Model file for the job. Use its own axes, mm. A direction names the side the tool comes from. Round coordinates to 2 decimals unless told otherwise and drop trailing zeros. Loops run counter-clockwise (first coordinate to the right, second up) from the corner with the lowest first, then second, coordinate; pieces in that order, holes last. Notation, with made-up numbers: M 42,80 L 50,80 A31 cw 50,113 Z; hole C -7.5,65.5 d10. An arc over 180 degrees is marked long. Answer in a Markdown table with one row per item.
from build123d import *

# Parameters (mm, degrees)
SKETCH1_W               = 55
SKETCH1_H               = 80
BOSS_EXTRUDE1_DEPTH     = 20
SKETCH2_W               = 49
SKETCH2_H               = 74
CUT_EXTRUDE1_DEPTH      = 17
SKETCH4_W               = 16
SKETCH4_H               = 12
BOSS_EXTRUDE2_DEPTH     = 40
SKETCH6_W               = 18
SKETCH6_H               = 20
CUT_EXTRUDE2_DEPTH      = 43
SKETCH5_W               = 5
SKETCH5_H               = 4
CUT_EXTRUDE3_DEPTH      = 15
SKETCH7_W               = 4.6
SKETCH7_H               = 8.6
CUT_EXTRUDE6_DEPTH      = 34
SKETCH9_W               = 3.9
SKETCH9_H               = 8.6
CUT_EXTRUDE7_DEPTH      = 17
SKETCH10_R              = 1
CUT_EXTRUDE8_DEPTH      = 3
SKETCH13_W              = 7
SKETCH13_H              = 18
BOSS_EXTRUDE3_DEPTH     = 7
CUT_EXTRUDE9_DEPTH      = 3
CUT_EXTRUDE9_DEPTH_BACK = 9
SKETCH14_W              = 12
SKETCH14_H              = 2


with BuildPart() as part:
    # Sketch1 → Boss-Extrude1 (new body)
    with BuildSketch(Plane(origin=(0, 0, 0), x_dir=(1, 0, 0), z_dir=(0, 1, 0))):
        Rectangle(SKETCH1_W, SKETCH1_H)
    extrude(amount=BOSS_EXTRUDE1_DEPTH)

    # Sketch2 → Cut-Extrude1 (cut)
    with BuildSketch(Plane(origin=(0, 20, 0), x_dir=(1, 0, 0), z_dir=(0, 1, 0))):
        Rectangle(SKETCH2_W, SKETCH2_H)
    extrude(amount=-CUT_EXTRUDE1_DEPTH, mode=Mode.SUBTRACT)

    # Sketch4 → Boss-Extrude2 (add)
    with BuildSketch(Plane(origin=(0, 20, 0), x_dir=(1, 0, 0), z_dir=(0, 1, 0))):
        with Locations((-35.5, 0)):
            Rectangle(SKETCH4_W, SKETCH4_H)
    extrude(amount=-BOSS_EXTRUDE2_DEPTH)

    # Sketch6 → Cut-Extrude2 (cut)
    with BuildSketch(Plane(origin=(0, 20, 0), x_dir=(1, 0, 0), z_dir=(0, 1, 0))):
        with Locations((-43.5, 0)):
            Rectangle(SKETCH6_W, SKETCH6_H)
    extrude(amount=-CUT_EXTRUDE2_DEPTH, mode=Mode.SUBTRACT)

    # Sketch5 → Cut-Extrude3 (cut)
    with BuildSketch(Plane.ZY.offset(43.5)):
        with Locations((0, -15)):
            Rectangle(SKETCH5_W, SKETCH5_H)
    extrude(amount=-CUT_EXTRUDE3_DEPTH, mode=Mode.SUBTRACT)

    # Sketch7 → Cut-Extrude6 (cut)
    with BuildSketch(Plane(origin=(0, 20, 0), x_dir=(1, 0, 0), z_dir=(0, 1, 0))):
        with Locations((-30.7, 0)):
            Rectangle(SKETCH7_W, SKETCH7_H)
    extrude(amount=-CUT_EXTRUDE6_DEPTH, mode=Mode.SUBTRACT)

    # Sketch9 → Cut-Extrude7 (cut)
    with BuildSketch(Plane(origin=(0, 20, 0), x_dir=(1, 0, 0), z_dir=(0, 1, 0))):
        with Locations((-26.45, 0)):
            Rectangle(SKETCH9_W, SKETCH9_H)
    extrude(amount=-CUT_EXTRUDE7_DEPTH, mode=Mode.SUBTRACT)

    # Sketch10 → Cut-Extrude8 (cut)
    with BuildSketch(Plane(origin=(0, 20, 0), x_dir=(1, 0, 0), z_dir=(0, 1, 0))):
        with Locations(Location((-26, -38.5, 0), (0, 0, 270))):
            Circle(SKETCH10_R)
        with Locations(Location((26, -38.5, 0), (0, 0, 270))):
            Circle(SKETCH10_R)
        with Locations(Location((26, 38.5, 0), (0, 0, 270))):
            Circle(SKETCH10_R)
        with Locations(Location((-26, 38.5, 0), (0, 0, 270))):
            Circle(SKETCH10_R)
    extrude(amount=-CUT_EXTRUDE8_DEPTH, mode=Mode.SUBTRACT)

    # Sketch13 → Boss-Extrude3 (add)
    with BuildSketch(Plane(origin=(0, 0, 0), x_dir=(-1, 0, 0), z_dir=(0, -1, 0))):
        with Locations((0, 20)):
            Rectangle(SKETCH13_W, SKETCH13_H)
        with Locations((0, -20)):
            Rectangle(SKETCH13_W, SKETCH13_H)
    extrude(amount=BOSS_EXTRUDE3_DEPTH)

    # Sketch14 → Cut-Extrude9 (cut, two sides: drawn at the far end of the back side and taken through both)
    with BuildSketch(Plane.ZY.offset(3.5).offset(-CUT_EXTRUDE9_DEPTH_BACK)):
        with Locations((-20, -3.5)):
            Rectangle(SKETCH14_W, SKETCH14_H)
        with Locations((20, -3.5)):
            Rectangle(SKETCH14_W, SKETCH14_H)
    extrude(amount=CUT_EXTRUDE9_DEPTH + CUT_EXTRUDE9_DEPTH_BACK, mode=Mode.SUBTRACT)


solid = part.part
1. Wall check: probe 1 along X at (y, z) = (18.6, 38.5); probe 2 along Z at (x, y) = (-26, 12.5); probe 3 along X at (y, z) = (4.5, -20.5). Give the ranges that are in metal, low to high.
Verdict:
| item | result |
|---|---|
| probe 1 | x = -27.5 to -27, -25 to 25, 27 to 27.5 |
| probe 2 | z = -40 to -4.3, 4.3 to 40 |
| probe 3 | x = -27.5 to -24.5, 24.5 to 27.5 |
2. Pin check, flat tips, straight feed: pin 1 (6 mm diameter, centred on x = 8, z = 24.5, fed in from -Y); pin 2 (10 mm diameter, centred on y = 14, z = 22, fed in from -X); pin 3 (7.5 mm diameter, centred on x = 1, z = -20.5, fed in from +Y). Stop position of each tip, or through.
Verdict:
| item | result |
|---|---|
| pin 1 | stops at y = 0 |
| pin 2 | stops at x = -27.5 |
| pin 3 | stops at y = 3 |
3. Saw through at A-A (y = -11). Write the cut outline in (x, z).
Verdict:
| item | result |
|---|---|
| outline | M -34.5,-6 L -27.5,-6 L -27.5,6 L -34.5,6 Z; hole M -33,-4.3 L -28.4,-4.3 L -28.4,4.3 L -33,4.3 Z |
4. Saw through at C-C (x = -23.5). Write the cut outline in (y, z).
Verdict:
| item | result |
|---|---|
| outline | M 0,-40 L 20,-40 L 20,-37 L 3,-37 L 3,37 L 20,37 L 20,40 L 0,40 Z |
5. Tool access for faces 1 (the flat face through (-3.5, -5, -20)), 2 (the flat face through (0, 12, -37)), 3 (the flat face through (0, -4.5, 20)), 4 (the flat face through (-27.5, 10, 23)), 5 (the flat face through (0, -3, 29)): list every direction of +Z, -Z, +X, -X, +Y, -Y with a clear straight run to the whole face (end or side of a thin tool).
Verdict:
| item | result |
|---|---|
| face 1 | +Z, -Z, -X, -Y |
| face 2 | +Y |
| face 3 | +X, -X |
| face 4 | +Z, -X, +Y, -Y |
| face 5 | +Z, +X, -X, -Y |
6. Mould opens along Y. For faces 6 (the flat face through (-26, 17, 38)), 7 (the flat face through (-33, 3, 0)), 8 (the flat face through (0, -4, 26)), 9 (the flat face through (0, -7, -20)) say: +Y half, -Y half, draft (parallel to the pull), parting line (faces both ways), or undercut.
Verdict:
| item | result |
|---|---|
| face 6 | +Y half |
| face 7 | draft |
| face 8 | undercut |
| face 9 | -Y half |
7. Saw through at D-D (z = 38.5). Write the cut outline in (x, y).
Verdict:
| item | result |
|---|---|
| outline | M -27.5,0 L 27.5,0 L 27.5,20 L 27,20 L 27,17 L 25,17 L 25,20 L -25,20 L -25,17 L -27,17 L -27,20 L -27.5,20 Z |
8. Saw through at B-B (z = -25). Write the cut outline in (x, y).
Verdict:
| item | result |
|---|---|
| outline | M -27.5,0 L -3.5,0 L -3.5,-2.5 L 3.5,-2.5 L 3.5,0 L 27.5,0 L 27.5,20 L 24.5,20 L 24.5,3 L -24.5,3 L -24.5,20 L -27.5,20 Z; M -3.5,-7 L 3.5,-7 L 3.5,-4.5 L -3.5,-4.5 Z |
